Source: CAD feature listing. Evaluate the final solid. Frame: model axes, mm. A direction names the side the tool comes from. Give positions to 0.01 mm unless a question says otherwise; leave off trailing zeros. Write each question's results on one line, items separated by ' | '. Start each with the question number.
Item 1: Line query: line 1 along X through (y, z) = (-19.5, -28); line 2 along X through (y, z) = (19, -107); line 3 along Y through (x, z) = (31, -71). Output: solid intervals per line, ascending.
Item 2: Mould query, pull axis Y, two halves, no side actions, for faces 1 (the flat face through (-50, 6, -15)), 2 (the flat face through (-53, 0, -30)), 3 (the flat face through (3, -62, -125)). Classes: released by +Y, released by -Y, zero draft, split by the parting line, or undercut.
Item 3: Contact query for flat-ended pins moving along their axis: pin 1 Ø3 at (x, z) = (-36.5, -75) entering from -Y; pin 2 Ø8 at (x, z) = (2.5, -14) entering from -Y; pin 3 Ø12 at (x, z) = (20, -25) entering from +Y. Output: stop coordinate, or through.
Item 4: Set-up query: faces 4 (the flat face through (2, -36, 0)), 5 (the flat face through (-51, -6, -15)). Return all of +Z, -Z, +X, -X, +Y, -Y with unobstructed straight access to the full face (end or side cutting, diameter ignored); none if empty.
```python
from build123d import *

# Parameters (mm, degrees)
SKETCH2_W                      = 112
SKETCH2_H                      = 102
BOSS_EXTRUDE1_DEPTH            = 125
BOSS_EXTRUDE1_TAPER            = -10
SKETCH3_W                      = 80
SKETCH3_H                      = 70
CUT_EXTRUDE1_DEPTH             = 125
CUT_EXTRUDE1_TAPER             = -10
CUT_EXTRUDE2_REACH             = 140.041
SKETCH5_W                      = 30
SKETCH5_H                      = 12
CUT_EXTRUDE2_DIRECTION_2_DEPTH = 10


with BuildPart() as part:
    # Sketch2 → Boss-Extrude1 (new body)
    with BuildSketch(Plane.XY):
        Rectangle(SKETCH2_W, SKETCH2_H)
    extrude(amount=-BOSS_EXTRUDE1_DEPTH, taper=BOSS_EXTRUDE1_TAPER)

    # Sketch3 → Cut-Extrude1 (cut)
    with BuildSketch(Plane(origin=(0, 0, 0), x_dir=(-1, 0, 0), z_dir=(0, 0, -1))):
        Rectangle(SKETCH3_W, SKETCH3_H)
    extrude(amount=CUT_EXTRUDE1_DEPTH, taper=CUT_EXTRUDE1_TAPER, mode=Mode.SUBTRACT)

    # Sketch5 → Cut-Extrude2 (cut, up to next)
    with BuildSketch(Plane(origin=(-60, 0, 0), x_dir=(0, 0, -1), z_dir=(1, 0, 0)), mode=Mode.PRIVATE) as cut_extrude2_sk1:
        with Locations((15, 0)):
            Rectangle(SKETCH5_W, SKETCH5_H)
    cut_extrude2_tool1 = extrude(cut_extrude2_sk1.sketch, amount=CUT_EXTRUDE2_REACH, mode=Mode.PRIVATE) & part.part
    add(cut_extrude2_tool1.solids().sort_by_distance((-60, 0, -15))[0], mode=Mode.SUBTRACT)

    # Sketch5 → Cut-Extrude2 direction 2 (cut)
    with BuildSketch(Plane(origin=(-60, 0, 0), x_dir=(0, 0, -1), z_dir=(1, 0, 0))):
        with Locations((15, 0)):
            Rectangle(SKETCH5_W, SKETCH5_H)
    extrude(amount=-CUT_EXTRUDE2_DIRECTION_2_DEPTH, mode=Mode.SUBTRACT)


solid = part.part
```
Evaluation:
1) line 1: x = -60.94 to -44.94, 44.94 to 60.94 | line 2: x = -74.87 to -58.87, 58.87 to 74.87 | line 3: y = -63.52 to -47.52, 47.52 to 63.52
2) face 1: undercut | face 2: undercut | face 3: zero draft
3) pin 1: stops at y = -64.49 | pin 2: stops at y = -54.17 | pin 3: stops at y = 56.47
4) face 4: +Z, +X, -X, +Y, -Y | face 5: +Z, -X
